from build123d import *

# Parameters (mm, degrees)
BOSS_EXTRUDE1_DEPTH      = 6.35
BOSS_EXTRUDE1_DEPTH_BACK = 6.35
SKETCH2_W                = 292.995908675
SKETCH2_H                = 3.175
CUT_EXTRUDE1_DEPTH       = 38.1
SKETCH3_W                = 146.05
SKETCH3_H                = 3.175
CUT_EXTRUDE2_DEPTH       = 38.1
CUT_EXTRUDE3_DEPTH       = 3.175
CUT_EXTRUDE4_DEPTH       = 3.175
CUT_EXTRUDE5_DEPTH       = 157.099
CUT_EXTRUDE6_DEPTH       = 339.217
CUT_EXTRUDE6_DEPTH_BACK  = 157.099
SKETCH9_W                = 50.8
SKETCH9_H                = 19.05
CUT_EXTRUDE7_DEPTH       = 21.59
SKETCH10_W               = 26.184999954
SKETCH10_H               = 36.77000012
CUT_EXTRUDE9_DEPTH       = 12.35
SKETCH11_W               = 3.53
SKETCH11_H               = 19.05
SKETCH11_W_2             = 0.965000048
CUT_EXTRUDE10_DEPTH      = 366.729881683
CUT_EXTRUDE11_DEPTH      = 5.08
SKETCH13_W               = 10.000000066
SKETCH13_H               = 4.999999906
CUT_EXTRUDE13_DEPTH      = 3.5


with BuildPart() as part:
    # Sketch1 → Boss-Extrude1 (new, two sides: drawn at the far end of the back side and taken through both)
    with BuildSketch(Plane(origin=(0, 0, 0), x_dir=(1, 0, 0), z_dir=(0, 1, 0)).offset(-BOSS_EXTRUDE1_DEPTH_BACK)):
        Polygon((-406.4, 0), (0, 0), (0, 146.05), (-152.4, 146.05), align=None)
    extrude(amount=BOSS_EXTRUDE1_DEPTH + BOSS_EXTRUDE1_DEPTH_BACK)

    # Sketch2 → Cut-Extrude1 (cut)
    with BuildSketch(Plane(origin=(-100.979614843, 0, -175.616721465), x_dir=(-0.8669063030575352, 0, 0.49847112425808277), z_dir=(-0.4984711242580827, 0, -0.8669063030575351))):
        with Locations((205.812767226, 4.7625)):
            Rectangle(SKETCH2_W, SKETCH2_H)
        with Locations((205.812767226, -4.7625)):
            Rectangle(SKETCH2_W, SKETCH2_H)
    extrude(amount=-CUT_EXTRUDE1_DEPTH, mode=Mode.SUBTRACT)

    # Sketch3 → Cut-Extrude2 (cut)
    with BuildSketch(Plane(origin=(0, 0, 0), x_dir=(0, 0, -1), z_dir=(1, 0, 0))):
        with Locations((73.025, 4.7625)):
            Rectangle(SKETCH3_W, SKETCH3_H)
        with Locations((73.025, -4.7625)):
            Rectangle(SKETCH3_W, SKETCH3_H)
    extrude(amount=-CUT_EXTRUDE2_DEPTH, mode=Mode.SUBTRACT)

    # Sketch4 → Cut-Extrude3 (cut)
    with BuildSketch(Plane(origin=(0, 6.35, 0), x_dir=(1, 0, 0), z_dir=(0, 1, 0))):
        Polygon((-133.408250166, 113.020869854), (-75.966284694, 146.05), (-152.4, 146.05), align=None)
    extrude(amount=-CUT_EXTRUDE3_DEPTH, mode=Mode.SUBTRACT)

    # Sketch5 → Cut-Extrude4 (cut)
    with BuildSketch(Plane.XZ.offset(6.35)):
        Polygon((-133.408250166, -113.020869854), (-75.966284694, -146.05), (-152.4, -146.05), align=None)
    extrude(amount=-CUT_EXTRUDE4_DEPTH, mode=Mode.SUBTRACT)

    # Sketch6 → Cut-Extrude5 (cut)
    with BuildSketch(Plane(origin=(0, 0, -146.05), x_dir=(-1, 0, 0), z_dir=(0, 0, -1))):
        Polygon((38.1, -3.175), (43.18, -3.175), (43.18, -6.35), (38.1, -6.35), (0, -6.35), (0, 6.35), (38.1, 6.35), (43.18, 6.35), (43.18, 3.175), (38.1, 3.175), (38.1, 1.5875), (35.56, 1.5875), (35.56, -1.5875), (38.1, -1.5875), align=None)
    extrude(amount=-CUT_EXTRUDE5_DEPTH, mode=Mode.SUBTRACT)

    # Sketch8 → Cut-Extrude6 (cut, two sides: drawn at the far end of the back side and taken through both)
    with BuildSketch(Plane(origin=(-51.420385157, 0, 29.566721465), x_dir=(0.49847112425808243, 0, 0.8669063030575355), z_dir=(-0.8669063030575355, 0, 0.49847112425808243)).offset(-CUT_EXTRUDE6_DEPTH_BACK)):
        Polygon((-164.478664898, 3.175), (-159.398664898, 3.175), (-159.398664898, 6.35), (-164.478664898, 6.35), (-202.578664898, 6.35), (-202.578664898, -6.35), (-164.478664898, -6.35), (-159.398664898, -6.35), (-159.398664898, -3.175), (-164.478664898, -3.175), (-164.478664898, -1.5875), (-167.018664898, -1.5875), (-167.018664898, 1.5875), (-164.478664898, 1.5875), align=None)
    extrude(amount=CUT_EXTRUDE6_DEPTH + CUT_EXTRUDE6_DEPTH_BACK, mode=Mode.SUBTRACT)

    # Sketch9 → Cut-Extrude7 (cut)
    with BuildSketch(Plane(origin=(0, 6.35, 0), x_dir=(1, 0, 0), z_dir=(0, 1, 0))):
        with Locations((-25.4, 136.525)):
            Rectangle(SKETCH9_W, SKETCH9_H)
    extrude(amount=-CUT_EXTRUDE7_DEPTH, mode=Mode.SUBTRACT)

    # Sketch10 → Cut-Extrude9 (cut)
    with BuildSketch(Plane(origin=(0, 6.35, 0), x_dir=(1, 0, 0), z_dir=(0, 1, 0))):
        with Locations((-64.857500025, 108.61499994)):
            Rectangle(SKETCH10_W, SKETCH10_H)
        Polygon((-44.680000048, 90.22999988), (-44.680000048, 127), (-50.8, 127), (-51.765000048, 127), (-51.765000048, 90.22999988), align=None)
    extrude(amount=-CUT_EXTRUDE9_DEPTH, mode=Mode.SUBTRACT)

    # Sketch11 → Cut-Extrude10 (cut, through all)
    with BuildSketch(Plane(origin=(0, 6.35, 0), x_dir=(1, 0, 0), z_dir=(0, 1, 0))):
        with Locations((-53.530000048, 136.525)):
            Rectangle(SKETCH11_W, SKETCH11_H)
        with Locations((-51.282500024, 136.525)):
            Rectangle(SKETCH11_W_2, SKETCH11_H)
    extrude(amount=-CUT_EXTRUDE10_DEPTH, mode=Mode.SUBTRACT)

    # Sketch12 → Cut-Extrude11 (cut)
    with BuildSketch(Plane(origin=(0, 6.35, 0), x_dir=(1, 0, 0), z_dir=(0, 1, 0))):
        Polygon((-103.350000002, 64.82999988), (-77.950000002, 90.22999988), (-77.950000002, 93.822102328), (-92.446051226, 79.326051104), (-104.958896043, 66.813206287), (-147.995170729, 50.489393917), (-253.068107346, 10.634854577), (-253.068107346, 7.62), align=None)
        Polygon((-74.357897554, 90.22999988), (-77.950000002, 90.22999988), (-103.350000002, 64.82999988), (-253.068107346, 7.62), (-253.068107346, 4.900877803), (-146.181884672, 45.744038959), (-113.564289699, 58.207812631), (-101.937140583, 62.65075685), (-88.853948778, 75.733948656), align=None)
    extrude(amount=-CUT_EXTRUDE11_DEPTH, mode=Mode.SUBTRACT)

    # Sketch13 → Cut-Extrude13 (cut)
    with BuildSketch(Plane.ZY.offset(44.680000048)):
        with Locations((-104.106, 0.175)):
            Rectangle(SKETCH13_W, SKETCH13_H)
    extrude(amount=-CUT_EXTRUDE13_DEPTH, mode=Mode.SUBTRACT)


solid = part.part
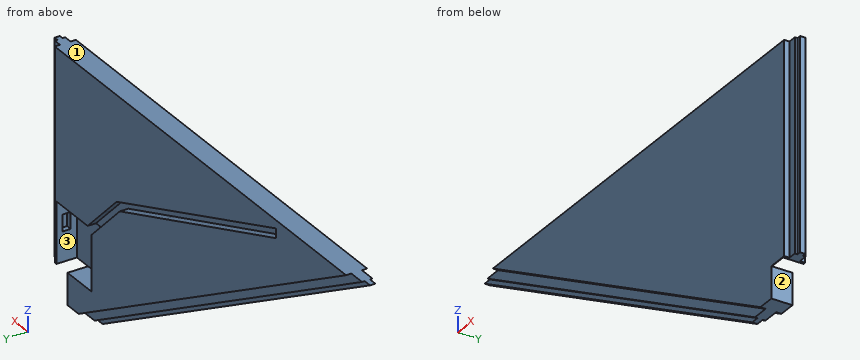
Verification items for the finished model (mm, model axes). Face numbers are marked on the shaded views. A direction names the side the tool comes from. Round coordinates to 2 decimals unless told otherwise and drop trailing zeros. Write each loop counter-clockwise with the first axis right and the second up, starting at its lowest first coordinate (ties: lowest second). Pieces come first, ordered by that corner, then holes.
(1) Section check D-D (x = -58). Enter the section's corners in (y, z).
Returned:
outline: (-6.35, -146.05) - (6.35, -146.05) - (6.35, -127) - (-6, -127) - (-6, -90.23) - (6.35, -90.23) - (6.35, 0) - (-6.35, 0) - close
(2) Access from +Z, -Z, +X, -X, +Y, -Y to the whole of each face (thin tool, end or side, straight path). Record for the marked faces 1, 2 and 3.
Returned:
face 1: +Z, +X, -X, +Y, -Y
face 2: -Z, +X, +Y, -Y
face 3: -Z, +Y
(3) Depth check by flat-ended pin: pin 1 Ø1.7 at (y, z) = (-3, -32) entering from +X; pin 2 Ø1 at (y, z) = (4.5, -60.5) entering from +X; pin 3 Ø10 at (x, z) = (-64, -109) entering from +Y. Enter the tip coordinate at first touch or a pass-through.
Returned:
pin 1: stops at x = -38.1
pin 2: stops at x = -43.18
pin 3: stops at y = -6
(4) Material ranges on line 1 (Z direction, x = -57.5, y = -1.75); line 2 (X direction, y = -4.25, z = -106); line 3 (Y direction, x = -211, z = -22.5), recorded low to high.
Returned:
line 1: z = -146.05 to -127, -90.23 to 0
line 2: x = -135.43 to -77.95, -44.68 to -43.18
line 3: y = -6.35 to 1.27
